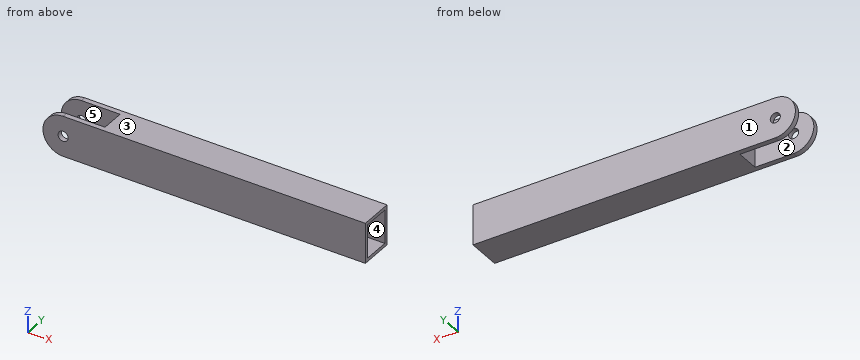
from build123d import *

# Parameters (mm, degrees)
SZKIC1_R                    = 1.5
DODANIE_WYCI_GNI_CIE1_DEPTH = 10
SZKIC2_W                    = 35
SZKIC2_H                    = 7
WYTNIJ_WYCI_GNI_CIE1_DEPTH  = 13
SZKIC3_W                    = 10
SZKIC3_H                    = 8
WYTNIJ_WYCI_GNI_CIE2_DEPTH  = 75


with BuildPart() as part:
    # Szkic1 → Dodanie-wyciągnięcie1 (new body)
    with BuildSketch(Plane(origin=(0, 0, 0), x_dir=(1, 0, 0), z_dir=(0, 1, 0))):
        with BuildLine():
            Line((0, 6), (90, 6))
            Line((90, 6), (90, -6))
            Line((90, -6), (0, -6))
            ThreePointArc((0, -6), (-6, 0), (0, 6))
        make_face()
        Circle(SZKIC1_R, mode=Mode.SUBTRACT)
    extrude(amount=DODANIE_WYCI_GNI_CIE1_DEPTH)

    # Szkic2 → Wytnij-wyciągnięcie1 (cut, through all)
    with BuildSketch(Plane(origin=(0, 0, -6), x_dir=(-1, 0, 0), z_dir=(0, 0, -1))):
        with Locations((6, 5)):
            Rectangle(SZKIC2_W, SZKIC2_H)
    extrude(amount=-WYTNIJ_WYCI_GNI_CIE1_DEPTH, mode=Mode.SUBTRACT)

    # Szkic3 → Wytnij-wyciągnięcie2 (cut)
    with BuildSketch(Plane(origin=(90, 0, 0), x_dir=(0, 0, -1), z_dir=(1, 0, 0))):
        with Locations((0, 5)):
            Rectangle(SZKIC3_W, SZKIC3_H)
    extrude(amount=-WYTNIJ_WYCI_GNI_CIE2_DEPTH, mode=Mode.SUBTRACT)


solid = part.part
Work out the finished part from the listing and answer in its coordinate system (mm). Face numbers are marked on the shaded views. A direction names the side the tool comes from. Round coordinates to 2 decimals unless told otherwise and drop trailing zeros. Loops run counter-clockwise (first coordinate to the right, second up) from the corner with the lowest first, then second, coordinate; pieces in that order, holes last. Notation, with made-up numbers: (-22, 3.25) - (12, 3.25) arc R31 cw to (12, 33.25) - close; hole circle Ø8 at (21.25, -35.5). An arc over 180 degrees is marked (long way). One line per item, written item: value.
Q1. Find section C-C on x = 43. Give the vertices of the cut face in (y, z), and give its area (3 significant figures).
Check values:
outline: (0, -6) - (10, -6) - (10, 6) - (0, 6) - close; hole (1, -5) - (9, -5) - (9, 5) - (1, 5) - close
area: 40.0 mm2
Q2. Find section A-A on z = 0. Give the vertices of the cut face in (x, y).
Check values:
outline: (-6, 0) - (-1.5, 0) - (-1.5, 1.5) - (-6, 1.5) - close; (-6, 8.5) - (-1.5, 8.5) - (-1.5, 10) - (-6, 10) - close; (1.5, 0) - (90, 0) - (90, 1) - (15, 1) - (15, 9) - (90, 9) - (90, 10) - (1.5, 10) - (1.5, 8.5) - (11.5, 8.5) - (11.5, 1.5) - (1.5, 1.5) - close
Q3. The mould has two halves that part along Z. Classify the marked faces 3, 4 and 5: +Z half, -Z half, draft (parallel to the pull), parting line (faces both ways), or undercut.
Check values:
face 3: +Z half
face 4: undercut
face 5: draft
Q4. Each of these flat-tipped pins is pushed along its axis until it touches: pin 1 Ø5 at (y, z) = (6, 0) entering from +X; pin 2 Ø3.5 at (y, z) = (5.5, -2) entering from -X. Where does it stop, or does it pass through?
Check values:
pin 1: x = 15
pin 2: x = 11.5
Q5. Straight lines are drawn through the part: probe 1 along X at (y, z) = (0.4, 0); probe 2 along Y at (x, z) = (0, 5); probe 3 along Y at (x, z) = (43, 4). For each, find the intervals that lie inside material, in ascending order.
Check values:
probe 1: -6 to -1.5, 1.5 to 90
probe 2: 0 to 1.5, 8.5 to 10
probe 3: 0 to 1, 9 to 10
Q6. Find section D-D on y = 5.25. Give the vertices of the cut face in (x, z).
Check values:
outline: (11.5, -6) - (90, -6) - (90, -5) - (15, -5) - (15, 5) - (90, 5) - (90, 6) - (11.5, 6) - close
Q7. Find section B-B on x = 10. Give the vertices of the cut face in (y, z), and give its area (3 significant figures).
Check values:
outline: (0, -6) - (1.5, -6) - (1.5, 6) - (0, 6) - close; (8.5, -6) - (10, -6) - (10, 6) - (8.5, 6) - close
area: 36.0 mm2
Q8. For the marked faces 1 and 2, determine the directions among +Z, -Z, +X, -X, +Y, -Y from which every point of the face is accessible in a straight line to the end or side of a thin tool.
Check values:
face 1: +Z, -Z, +X, -X, +Y
face 2: +Z, -Z, -X
